Geometry check sheet. Reference: the model listing, model coordinates, mm. Face numbers are marked on the shaded views. A direction names the side the tool comes from. Round coordinates to 2 decimals unless told otherwise and drop trailing zeros. Order: outer loops, then holes, each group sorted by start corner. A loop starts at its lowest first (then second) coordinate and runs counter-clockwise, first axis right, second up. Notation, with made-up numbers: (53, 84) - (78, 84) arc R19 cw to (78, 112) - close; hole circle Ø9 at (-12, 28.25). An arc over 180 degrees is marked (long way). Return JSON: item names as keys, results as strings. Group by question number.
Q1. Tool access check on the marked faces 1 and 2. Record the directions out of +Z, -Z, +X, -X, +Y, -Y that give a thin tool (end or side, any length) a straight path to the whole face; none if there is none.
Q2. Sectioned sample at A-A, the plane x = 0. Give the number of separate pieces and of enclosed holes in the cut face, then the cut area to 3 significant figures.
Q3. Sectioned sample at D-D, the plane y = -7.5. Record the cut outline in (x, z) (3 decimals), then the cut area to 3 significant figures.
Q4. Sectioned sample at C-C, the plane x = -28.1. Record the cut outline in (y, z) (3 decimals).
Q5. Material ranges on line 1 along Y through (x, z) = (-28.1, 10.2); line 2 along Y through (x, z) = (30.5, -2.75) (3 decimals); line 3 along Z through (x, y) = (-29, 3.5) (3 decimals), recorded low to high.
Q6. Draft check along Y on the marked faces 3, 4 and 5. Enter one of: pulls with the +Y half, pulls with the -Y half, needs draft (parallel to the pull), parting line crosses it, or undercut.
Q7. Gauge pin test, flat end, axial feed: pin 1 Ø7 at (x, y) = (0, 25.4) entering from -Z (3 decimals). Record the tip position at first contact, or that the pin passes through.
Q8. Sectioned sample at B-B, the plane z = -5. Record the cut outline in (x, y) (3 decimals), then the cut area to 3 significant figures.
```python
from build123d import *

# Parameters (mm, degrees)
SKETCH1_W                                       = 76.2
SKETCH1_H                                       = 76.2
BOSS_EXTRUDE1_DEPTH                             = 12.7
SKETCH2_W                                       = 19.05
SKETCH2_H                                       = 69.85
CUT_EXTRUDE1_DEPTH                              = 77.2
SKETCH4_R                                       = 9.75
SKETCH4_R_2                                     = 2.2
SKETCH4_R_3                                     = 2.368967754
SKETCH4_R_4                                     = 2.114206927
SKETCH4_R_5                                     = 2.315385773
SKETCH4_R_6                                     = 1.799630575
CUT_EXTRUDE2_DEPTH                              = 26.4
CBORE_FOR_M6_SOCKET_HEAD_CAP_SCREW1_D           = 6.4
CBORE_FOR_M6_SOCKET_HEAD_CAP_SCREW1_CBORE_D     = 11
CBORE_FOR_M6_SOCKET_HEAD_CAP_SCREW1_CBORE_DEPTH = 6.4
CUT_EXTRUDE3_REACH                              = 27.4
SKETCH8_R                                       = 3.81
CBORE_FOR_M5_SOCKET_HEAD_CAP_SCREW3_D           = 5.3
CBORE_FOR_M5_SOCKET_HEAD_CAP_SCREW3_CBORE_D     = 10
CBORE_FOR_M5_SOCKET_HEAD_CAP_SCREW3_CBORE_DEPTH = 5.4


with BuildPart() as part:
    # Sketch1 → Boss-Extrude1 (new body, symmetric)
    with BuildSketch(Plane.XY):
        Rectangle(SKETCH1_W, SKETCH1_H)
    extrude(amount=BOSS_EXTRUDE1_DEPTH, both=True)

    # Sketch2 → Cut-Extrude1 (cut, through all)
    with BuildSketch(Plane(origin=(38.1, 0, 0), x_dir=(0, 0, -1), z_dir=(1, 0, 0))):
        Rectangle(SKETCH2_W, SKETCH2_H)
    extrude(amount=-CUT_EXTRUDE1_DEPTH, mode=Mode.SUBTRACT)

    # Sketch4 → Cut-Extrude2 (cut, through all)
    with BuildSketch(Plane.XY.offset(12.7)):
        Circle(SKETCH4_R)
        with Locations((0, 25.4)):
            Circle(SKETCH4_R_2)
        with Locations((-28.1, 28.1)):
            Circle(SKETCH4_R_3)
        with Locations((28.1, 28.1)):
            Circle(SKETCH4_R_4)
        with Locations((-28.1, -28.1)):
            Circle(SKETCH4_R_5)
        with Locations((28.1, -28.1)):
            Circle(SKETCH4_R_6)
        with Locations((0, -25.4)):
            Circle(SKETCH4_R_2)
    extrude(amount=-CUT_EXTRUDE2_DEPTH, mode=Mode.SUBTRACT)

    # CBORE for M6 Socket Head Cap Screw1 (through all)
    with Locations(Plane.XY.offset(12.7)):
        with Locations((-28.1, 28.1), (28.1, 28.1), (28.1, -28.1), (-28.1, -28.1)):
            CounterBoreHole(CBORE_FOR_M6_SOCKET_HEAD_CAP_SCREW1_D / 2, CBORE_FOR_M6_SOCKET_HEAD_CAP_SCREW1_CBORE_D / 2, CBORE_FOR_M6_SOCKET_HEAD_CAP_SCREW1_CBORE_DEPTH)

    # Sketch8 → Cut-Extrude3 (cut, up to next)
    with BuildSketch(Plane(origin=(0, 0, -12.7), x_dir=(-1, 0, 0), z_dir=(0, 0, -1)), mode=Mode.PRIVATE) as cut_extrude3_sk1:
        with Locations((0, 25.4)):
            Circle(SKETCH8_R)
    cut_extrude3_tool1 = extrude(cut_extrude3_sk1.sketch, amount=-CUT_EXTRUDE3_REACH, mode=Mode.PRIVATE) & part.part
    add(cut_extrude3_tool1.solids().sort_by_distance((0, 25.4, -12.7))[0], mode=Mode.SUBTRACT)
    # Sketch8 → Cut-Extrude3 (cut, up to next)
    with BuildSketch(Plane(origin=(0, 0, -12.7), x_dir=(-1, 0, 0), z_dir=(0, 0, -1)), mode=Mode.PRIVATE) as cut_extrude3_sk2:
        with Locations((0, -25.4)):
            Circle(SKETCH8_R)
    cut_extrude3_tool2 = extrude(cut_extrude3_sk2.sketch, amount=-CUT_EXTRUDE3_REACH, mode=Mode.PRIVATE) & part.part
    add(cut_extrude3_tool2.solids().sort_by_distance((0, -25.4, -12.7))[0], mode=Mode.SUBTRACT)

    # CBORE for M5 Socket Head Cap Screw3 (through all)
    with Locations(Plane(origin=(0, 0, -12.7), x_dir=(-1, 0, 0), z_dir=(0, 0, -1))):
        with Locations((0, -25.4), (0, 25.4)):
            CounterBoreHole(CBORE_FOR_M5_SOCKET_HEAD_CAP_SCREW3_D / 2, CBORE_FOR_M5_SOCKET_HEAD_CAP_SCREW3_CBORE_D / 2, CBORE_FOR_M5_SOCKET_HEAD_CAP_SCREW3_CBORE_DEPTH)


solid = part.part
```
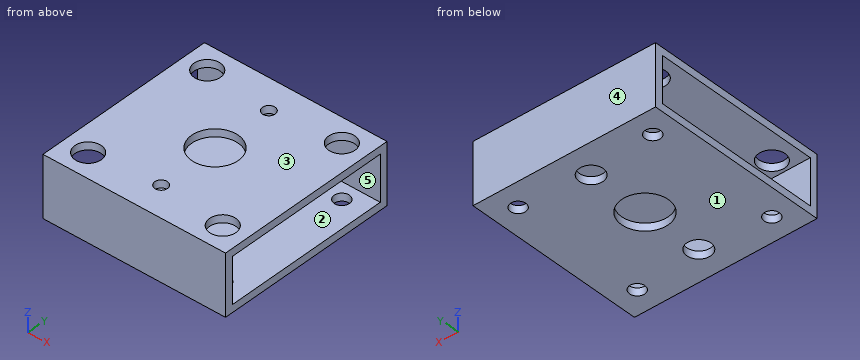
Reply:
{
 "1": {"face 1": "-Z, +X, -X, +Y, -Y", "face 2": "+X, -X"},
 "2": {"separate pieces": "6", "enclosed holes": "0", "area": "384 mm^2"},
 "3": {"outline": "(-38.1, -12.7) - (-6.23, -12.7) - (-6.23, -9.525) - (-38.1, -9.525) - close; (-38.1, 9.525) - (-6.23, 9.525) - (-6.23, 12.7) - (-38.1, 12.7) - close; (6.23, -12.7) - (38.1, -12.7) - (38.1, -9.525) - (6.23, -9.525) - close; (6.23, 9.525) - (38.1, 9.525) - (38.1, 12.7) - (6.23, 12.7) - close", "area": "405 mm^2"},
 "4": {"outline": "(-38.1, -12.7) - (-31.3, -12.7) - (-31.3, -9.525) - (-34.925, -9.525) - (-34.925, 9.525) - (-33.6, 9.525) - (-33.6, 12.7) - (-38.1, 12.7) - close; (-24.9, -12.7) - (24.9, -12.7) - (24.9, -9.525) - (-24.9, -9.525) - close; (-22.6, 9.525) - (22.6, 9.525) - (22.6, 12.7) - (-22.6, 12.7) - close; (31.3, -12.7) - (38.1, -12.7) - (38.1, 12.7) - (33.6, 12.7) - (33.6, 9.525) - (34.925, 9.525) - (34.925, -9.525) - (31.3, -9.525) - close"},
 "5": {"line 1": "-38.1 to -33.6, -22.6 to 22.6, 33.6 to 38.1", "line 2": "-38.1 to -34.925, 34.925 to 38.1", "line 3": "-12.7 to -9.525, 9.525 to 12.7"},
 "6": {"face 3": "needs draft", "face 4": "pulls with the +Y half", "face 5": "undercut"},
 "7": {"pin 1": "z = 9.525"},
 "8": {"outline": "(-38.1, -38.1) - (38.1, -38.1) - (38.1, -34.925) - (-38.1, -34.925) - close; (-38.1, 34.925) - (38.1, 34.925) - (38.1, 38.1) - (-38.1, 38.1) - close", "area": "484 mm^2"}
}
